Part model, mm, in its own coordinate system. Face numbers are marked on the shaded views. A direction names the side the tool comes from. Round coordinates to 2 decimals unless told otherwise and drop trailing zeros. Write each loop counter-clockwise with the first axis right and the second up, starting at its lowest first coordinate (ties: lowest second). Pieces come first, ordered by that corner, then holes.
1) Flat gauge pins, fed straight in: pin 1 (0.6 mm diameter, centred on x = -22, y = -19, fed in from +Z) (3 decimals); pin 2 (6 mm diameter, centred on y = -32.5, z = -23, fed in from -X); pin 3 (7.5 mm diameter, centred on y = -14, z = -24, fed in from -X) (3 decimals). Where does each tip first touch, or does it go through?
2) Which spindle directions (+Z, -Z, +X, -X, +Y, -Y) get a long thin tool onto all of the face, cutting with end or side? Do the marked faces 3, 4 and 5. Say none if no direction does.
3) Pull direction X, two halves, no side cores. Call the marked faces 1 and 2: +X half, -X half, draft (parallel to the pull), parting line (faces both ways), or undercut.
4) Saw through at B-B on z = -23. Count the separate pieces of the cut face and the enclosed holes in it, and give its area (3 significant figures).
5) Drill centre lines: L1, parallel to X at y = -21, z = -23; L2, parallel to X at y = -23.5, z = -19.5; L3, parallel to X at y = -15.5, z = -14. Where is each one in solid material? Low to high.
6) Saw through at D-D on x = -9. Write the cut outline in (y, z) (3 decimals), and give its area (3 significant figures).
7) Saw through at A-A on z = -30. Write the cut outline in (x, y), and give its area (3 significant figures).
```python
from build123d import *

# Parameters (mm, degrees)
F0_W     = 38.1
F0_H     = 38.1
F1_DEPTH = 38.1
F5_DEPTH = 38.1
F7_DEPTH = 38.1
F8_W     = 7.62
F8_H     = 25.4
F9_DEPTH = 38.1


with BuildPart() as f1:
    # F0 (on Front) → F1 (new body)
    with BuildSketch(Plane.XZ):
        with Locations((-19.05, -19.05)):
            Rectangle(F0_W, F0_H)
    extrude(amount=F1_DEPTH)

    # F4 (on offset) → F5 (cut)
    with BuildSketch(Plane.YZ.offset(-38.1)):
        Polygon((-25.4, -38.1), (-12.7, -38.1), (-19.05, -22.225), align=None)
        Polygon((-11.43, -22.225), (-6.35, 0), (-31.75, 0), (-26.67, -22.225), (-21.59, -9.525), (-16.51, -9.525), align=None)
        Polygon((-31.75, -38.1), (-38.1, 0), (-38.1, -38.1), align=None)
        Polygon((0, -38.1), (0, 0), (-6.35, -38.1), align=None)
    extrude(amount=F5_DEPTH, mode=Mode.SUBTRACT)

    # F6 (on offset) → F7 (cut)
    with BuildSketch(Plane.XZ.offset(38.1)):
        Polygon((-26.67, -15.875), (-31.75, -38.1), (-6.35, -38.1), (-11.43, -15.875), (-16.51, -28.575), (-21.59, -28.575), align=None)
        Polygon((-12.7, 0), (-25.4, 0), (-19.05, -15.875), align=None)
        Polygon((-6.35, 0), (0, -38.1), (0, 0), align=None)
        Polygon((-38.1, 0), (-38.1, -38.1), (-31.75, 0), align=None)
    extrude(amount=-F7_DEPTH, mode=Mode.SUBTRACT)

    # F8 (on Top) → F9 (cut)
    with BuildSketch(Plane.XY):
        with Locations((-11.43, -12.7)):
            Rectangle(F8_W, F8_H)
        Polygon((-30.48, -38.1), (-22.86, -38.1), (-22.648146, -12.7), (-30.48, -12.7), align=None)
    extrude(amount=-F9_DEPTH, mode=Mode.SUBTRACT)


solid = f1.part
```
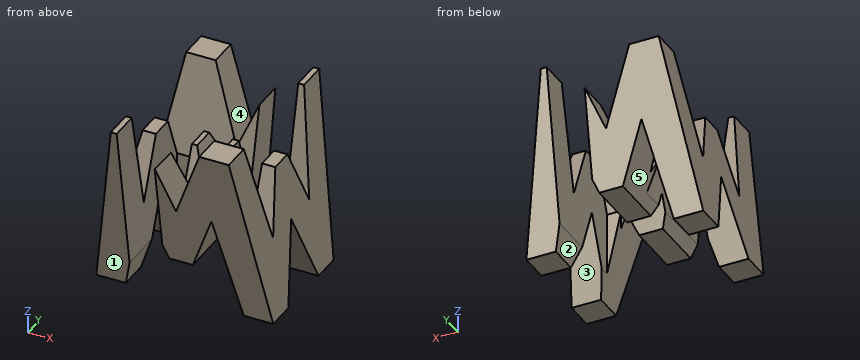
Completed:
1. pin 1: stops at z = -9.525
1. pin 2: stops at x = -36.08
1. pin 3: stops at x = -36.375
2. face 3: -Z, +X, -X
2. face 4: +Z, +Y, -Y
2. face 5: -Z, +Y, -Y
3. face 1: draft
3. face 2: undercut
4. separate pieces: 6
4. enclosed holes: 0
4. area: 585 mm2
5. L1: x = -35.58 to -30.48, -22.72 to -15.24, -7.62 to -2.52
5. L2: x = -35 to -30.48, -22.74 to -15.24, -7.62 to -3.1
5. L3: x = -34.08 to -30.48, -22.67 to -19.8, -18.3 to -15.24, -7.62 to -4.02
6. outline: (-38.1, 0) - (-33.682, -26.506) - (-25.4, -26.506) - (-25.4, -19.05) - (-26.67, -22.225) - (-31.75, 0) - close
6. area: 195 mm2
7. outline: (-36.75, -33.1) - (-30.48, -33.1) - (-30.48, -22.16) - (-36.75, -22.16) - close; (-36.75, -15.94) - (-30.48, -15.94) - (-30.48, -12.7) - (-29.9, -12.7) - (-29.9, -5) - (-36.75, -5) - close; (-8.2, -33.1) - (-1.35, -33.1) - (-1.35, -22.16) - (-7.62, -22.16) - (-7.62, -25.4) - (-8.2, -25.4) - close; (-7.62, -15.94) - (-1.35, -15.94) - (-1.35, -5) - (-7.62, -5) - close
7. area: 283 mm2
